Can you work these out from the model? Positions are in its coordinate system, mm. Face numbers are marked on the shaded views. A direction names the side the tool comes from. Round coordinates to 2 decimals unless told otherwise and drop trailing zeros. Loops run counter-clockwise (first coordinate to the right, second up) from the corner with the lowest first, then second, coordinate; pieces in that order, holes last.
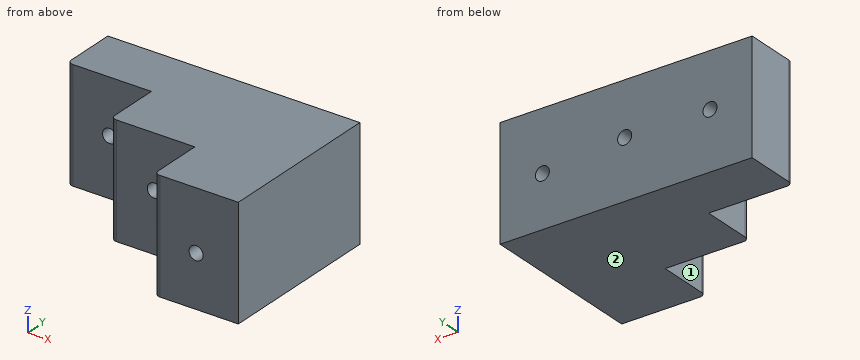
from build123d import *

# Parameters (mm, degrees)
F1_DEPTH = 400
F2_R     = 20
F4_R     = 25
F5_DEPTH = 200.001
F6_R     = 25
F7_DEPTH = 400.001
F8_R     = 25
F9_DEPTH = 600.001


with BuildPart() as f1:
    # F0 (on Top) → F1 (new body)
    with BuildSketch(Plane.XY):
        Polygon((900, 0), (0, 0), (0, -200), (300, -200), (300, -400), (600, -400), (600, -600), (900, -600), align=None)
    extrude(amount=F1_DEPTH)

    # F2
    f2_edges = [f1.edges().sort_by_distance(p)[0] for p in [
        (600, -600, 200),
        (300, -400, 200),
        (0, -200, 200),
    ]]
    fillet(f2_edges, radius=F2_R)

    # F4 (on face) → F5 (cut, through all)
    with BuildSketch(Plane.XZ.offset(200)):
        with Locations((150.4388, 206.492081)):
            Circle(F4_R)
    extrude(amount=-F5_DEPTH, mode=Mode.SUBTRACT)

    # F6 (on face) → F7 (cut, through all)
    with BuildSketch(Plane.XZ.offset(400)):
        with Locations((455.119699, 210.518703)):
            Circle(F6_R)
    extrude(amount=-F7_DEPTH, mode=Mode.SUBTRACT)

    # F8 (on face) → F9 (cut, through all)
    with BuildSketch(Plane.XZ.offset(600)):
        with Locations((749.062896, 185.016781)):
            Circle(F8_R)
    extrude(amount=-F9_DEPTH, mode=Mode.SUBTRACT)


solid = f1.part
(1) If we section it at D-D, the plane x = 211.5: List the corners of the cut face in (y, z) for me.
Worked answers:
outline: (-200, 0) - (0, 0) - (0, 400) - (-200, 400) - close
(2) Will these pins go through, and if not, where does the flat tip stop? P1, Ø6, axis at y = -230.5, z = 292, coming from the -X side; P2, Ø6, axis at x = 315, z = 200.5, coming from the -Y side; P3, Ø1.5, axis at x = 503.5, z = 51.5, coming from the -Y side.
Worked answers:
P1: stops at x = 300
P2: stops at y = -399.9
P3: stops at y = -400
(3) For the marked faces 1 and 2, which set-ups out of +Z, -Z, +X, -X, +Y, -Y let a thin tool reach every point of the face, with its end or its side?
Worked answers:
face 1: +Z, -Z, -X, -Y
face 2: -Z, +X, -X, +Y, -Y
(4) If we section it at B-B, the plane y = -86: List the corners of the cut face in (x, z) for me, then the cut area to 3 significant figures.
Worked answers:
outline: (0, 0) - (900, 0) - (900, 400) - (0, 400) - close; hole circle Ø50 at (150.44, 206.49); hole circle Ø50 at (455.12, 210.52); hole circle Ø50 at (749.06, 185.02)
area: 354,000 mm2
(5) If I drill on line 1 (X direction, y = -443, z = 49); line 2 (Y direction, x = 92, z = 349.5); line 3 (X direction, y = -312, z = 358), over which ranges is the centre line in solid material (lowest first)?
Worked answers:
line 1: x = 600 to 900
line 2: y = -200 to 0
line 3: x = 300 to 900
(6) If we section it at A-A, the plane x = 470: List the corners of the cut face in (y, z) for me.
Worked answers:
outline: (-400, 0) - (0, 0) - (0, 190.43) - (-400, 190.43) - close; (-400, 230.61) - (0, 230.61) - (0, 400) - (-400, 400) - close
(7) If we section it at C-C, the plane z = 334: List the corners of the cut face in (x, y) for me.
Worked answers:
outline: (0, -180) arc R20 ccw to (20, -200) - (300, -200) - (300, -380) arc R20 ccw to (320, -400) - (600, -400) - (600, -580) arc R20 ccw to (620, -600) - (900, -600) - (900, 0) - (0, 0) - close
